Autodesk Inventor part; units mm, degrees
ref_plane "YZ Plane" through (0, 0, 0) normal (1, 0, 0) x (0, 1, 0)
ref_plane "XZ Plane" through (0, 0, 0) normal (0, 1, 0) x (-1, 0, 0)
ref_plane "XY Plane" through (0, 0, 0) normal (0, 0, 1) x (1, 0, 0)
sketch "Sketch1" plane through (0, 0, 0) normal (0, 1, 0) x (-1, 0, 0)
  circle A0 centre (-3.2101, 3.6478) radius 9.5
  point P0 (0, 0)
  dimension "d0" = 19
extrude "Extrusion1" add sketch "Sketch1" along normal blind 5
chamfer "Chamfer1" distance 0.5 distance2 5 1 edges at (12.7101, 0, 3.6478) measured on face at (4.333, 0, 5.8992)
sketch "Sketch2" plane through (3.2101, 0, 3.6478) normal (0, -1, 0) x (1, 0, 0)
  circle A0 centre (0, 0) radius 5
  point P0 (-3.2101, -3.6478)
  dimension "d6" = 10
extrude "Extrusion2" cut sketch "Sketch2" against normal blind 5
properties part number "kop"
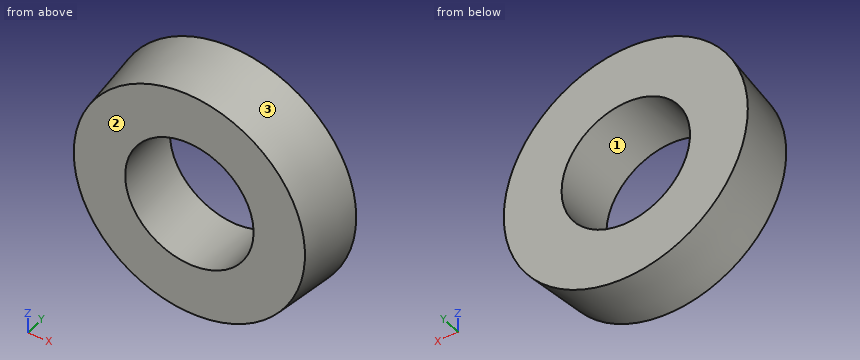
Verification items for the finished model (mm, model axes). Face numbers are marked on the shaded views. Give positions to 0.01 mm unless a question says otherwise; leave off trailing zeros. Loops run counter-clockwise (first coordinate to the right, second up) from the corner with the lowest first, then second, coordinate; pieces in that order, holes last.
1. Thickness scan on line 1 (X direction, y = 1.45, z = 7); line 2 (X direction, y = 2.15, z = 6.75); line 3 (Z direction, x = 7.5, y = 4.75). Record the ranges inside material, lowest first.
2. Mould release check, pull along X, two halves, no side actions. Record for the marked faces 1, 2 and 3: released by +X, released by -X, zero draft, split by the parting line, or undercut.
3. Section check A-A, the plane y = 0.7. Enter the section's corners in (x, z).
4. Go/stop test with flat-tipped pins: pin 1 Ø2 at (x, z) = (2.5, 0) entering from +Y; pin 2 Ø3 at (y, z) = (2.5, -1) entering from -X; pin 3 Ø1 at (y, z) = (2, -2) entering from +X; pin 4 Ø1.5 at (y, z) = (3, 9) entering from +X. Record where each tip stops, or that it passes through.
5. Section check B-B, the plane y = 4.35. Enter the section's corners in (x, z) (3 decimals), then the cut area to 3 significant figures.
Geometry says:
1. line 1: x = -5.3 to -0.5, 6.92 to 11.72
1. line 2: x = -5.47 to -0.71, 7.13 to 11.89
1. line 3: z = -4.8 to 1.08, 6.22 to 12.1
2. face 1: undercut
2. face 2: zero draft
2. face 3: split by the parting line
3. outline: circle Ø18.14 at (3.21, 3.65); hole circle Ø10 at (3.21, 3.65)
4. pin 1: passes through
4. pin 2: stops at x = -5.51
4. pin 3: stops at x = 10.84
4. pin 4: stops at x = 11.3
5. outline: circle Ø18.87 at (3.21, 3.648); hole circle Ø10 at (3.21, 3.648)
5. area: 201 mm2
